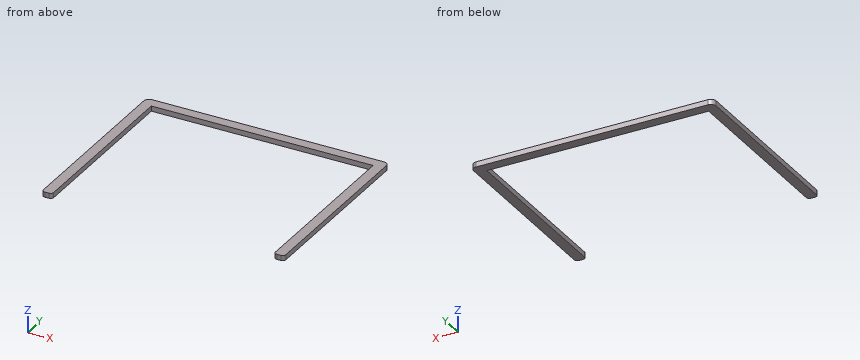
```python
from build123d import *

# Parameters (mm, degrees)
F1_DEPTH = 5


with BuildPart() as f1:
    # F0 (on Top) → F1 (new body)
    with BuildSketch(Plane.XY):
        with BuildLine():
            Line((-107.5, 87.5), (107.5, 87.5))
            Line((107.5, 87.5), (107.5, -84.516405))
            ThreePointArc((107.5, -84.516405), (108.372872, -86.631901), (110.483551, -87.516359))
            Line((110.483551, -87.516359), (114.483551, -87.538292))
            ThreePointArc((114.483551, -87.538292), (116.615497, -86.665465), (117.5, -84.538337))
            Line((117.5, -84.538337), (117.5, 92.5))
            ThreePointArc((117.5, 92.5), (116.035534, 96.035534), (112.5, 97.5))
            Line((112.5, 97.5), (-112.5, 97.5))
            ThreePointArc((-112.5, 97.5), (-116.035534, 96.035534), (-117.5, 92.5))
            Line((-117.5, 92.5), (-117.5, -84.461572))
            ThreePointArc((-117.5, -84.461572), (-116.627128, -86.577069), (-114.516449, -87.461527))
            Line((-114.516449, -87.461527), (-110.516449, -87.48346))
            ThreePointArc((-110.516449, -87.48346), (-108.384503, -86.610633), (-107.5, -84.483505))
            Line((-107.5, -84.483505), (-107.5, 87.5))
        make_face()
    extrude(amount=F1_DEPTH)


solid = f1.part
```
The listing builds one solid part. Answer for the finished solid, in the listing's coordinates (mm). Give positions to 0.01 mm unless a question says otherwise; leave off trailing zeros. Loops run counter-clockwise (first coordinate to the right, second up) from the corner with the lowest first, then second, coordinate; pieces in that order, holes last. Notation, with made-up numbers: (73.5, 11) - (95.5, 11) arc R24 ccw to (95.5, 38) - close; hole circle Ø7 at (-33, 0). An arc over 180 degrees is marked (long way). Return JSON: item names as keys, results as strings. Group by question number.
1. Straight lines are drawn through the part: line 1 (X direction, y = 27, z = 0.55); line 2 (Y direction, x = 86, z = 0.8). For each, find the intervals that lie inside material, in ascending order. Write a range as [from, to].
2. Find section A-A (y = -36). Write down the section's boundary in (x, z).
3. Find section C-C (x = 65.5). Write down the section's boundary in (y, z), then the cut area to 3 significant figures.
4. Find section B-B (z = 1.9). Write down the section's boundary in (x, y).
Verdict:
{
 "1": {"line 1": "x = [-117.5, -107.5], [107.5, 117.5]", "line 2": "y = [87.5, 97.5]"},
 "2": {"outline": "(-117.5, 0) - (-107.5, 0) - (-107.5, 5) - (-117.5, 5) - close; (107.5, 0) - (117.5, 0) - (117.5, 5) - (107.5, 5) - close"},
 "3": {"outline": "(87.5, 0) - (97.5, 0) - (97.5, 5) - (87.5, 5) - close", "area": "50.0 mm^2"},
 "4": {"outline": "(-117.5, -84.46) arc R3 ccw to (-114.52, -87.46) - (-110.52, -87.48) arc R3 ccw to (-107.5, -84.48) - (-107.5, 87.5) - (107.5, 87.5) - (107.5, -84.52) arc R3 ccw to (110.48, -87.52) - (114.48, -87.54) arc R3 ccw to (117.5, -84.54) - (117.5, 92.5) arc R5 ccw to (112.5, 97.5) - (-112.5, 97.5) arc R5 ccw to (-117.5, 92.5) - close"}
}
